Verification items for the finished model (mm, model axes). A direction names the side the tool comes from. Give positions to 0.01 mm unless a question says otherwise; leave off trailing zeros. Order: outer loops, then holes, each group sorted by start corner. A loop starts at its lowest first (then second) coordinate and runs counter-clockwise, first axis right, second up. Notation, with made-up numbers: (55.25, 0) -> (110.25, 0) arc R20 cw to (110.25, 33) -> close; hole circle Ø4 at (-6.75, 59). An arc over 180 degrees is marked (long way). One line per question, with ' | ' between items. Start each with the question number.
Q1. Section check A-A on x = 720. Record the cut outline in (y, z).
Q2. Access from +Z, -Z, +X, -X, +Y, -Y to the whole of each face (thin tool, end or side, straight path). Record for faces 3 (the flat face through (325.712, 4.93, -866.605)), 4 (the flat face through (869.54, 4.93, -1019.48)).
Q3. Go/stop test with flat-tipped pins: pin 1 (3 mm diameter, centred on x = 353.5, y = 7.5, fed in from +Z); pin 2 (5 mm diameter, centred on y = 4.5, z = -890.5, fed in from +X); pin 3 (6 mm diameter, centred on x = 1178, y = 9, fed in from -Z). Record where each tip stops, or that it passes through.
Q4. Section check D-D on x = 347. Record the cut outline in (y, z).
Q5. Material ranges on probe 1 along X at (y, z) = (7, -1119); probe 2 along X at (y, z) = (1.75, -945); probe 3 along Z at (x, y) = (1042, 5), recorded low to high. Write a range as [from, to].
Q6. Section check B-B on z = -682. Record the cut outline in (x, y).
Q7. Mould release check, pull along Z, two halves, no side actions. Record for faces 1 (the flat face through (745.285, 4.93, -1322.039)), 2 (the flat face through (611.047, 4.93, -1098.128)): released by +Z, released by -Z, zero draft, split by the parting line, or undercut.
Q8. Section check C-C on y = 7.25. Give the number of separate pieces and of enclosed holes in the cut face, plus the area to 3 significant figures.
from build123d import *

# Parameters (mm, degrees)
BOSS_EXTRUDE1_DEPTH = 10


with BuildPart() as part:
    # Sketch1 → Boss-Extrude1 (new body)
    with BuildSketch(Plane(origin=(0, 0, 0), x_dir=(1, 0, 0), z_dir=(0, 1, 0))):
        Polygon((784.987851723, 398.007183844), (785.000571871, 709.000734601), (783.999038632, 709.000734601), (648.95430554, 576.00627914), (204.012861183, 736.515465829), (389.346795443, 804.38206818), (260.269155542, 930.594602451), (438.985812263, 917.017059796), (281.997531244, 1251.994529906), (546.997134557, 1127.998293592), (540.820297596, 1358.942378927), (694.484658499, 1184.98269214), (797.527155209, 1462.988304378), (901.507891553, 1184.98269214), (1055.994737963, 1359.007597162), (1049.481640439, 1127.998293592), (1313.995431768, 1251.994529906), (1156.991756683, 916.99500763), (1334.998347933, 930.999939378), (1205.935810073, 803.988718502), (1391.001934492, 736.990931112), (946.559511347, 576.00627914), (810.545996287, 709.000734601), (809.987230906, 398.007183844), align=None)
        Polygon((768.211437064, 725.031722001), (643.992624095, 601.960316667), (269.679365999, 736.990931112), (486.122884579, 816.249412651), (530.047300467, 725.031722001), align=None, mode=Mode.SUBTRACT)
        Polygon((826.995686835, 725.031722001), (952.513065316, 601.960316667), (1325.302227186, 736.990931112), (1109.467295774, 816.249412651), (1065.831329223, 725.031722001), align=None, mode=Mode.SUBTRACT)
        Polygon((826.995686835, 747.043809063), (1052.054612149, 747.043809063), (1088.054253232, 823.06470125), (953.479995281, 872.126355119), align=None, mode=Mode.SUBTRACT)
        Polygon((767.95234015, 747.043809063), (543.908716076, 747.043809063), (507.909790164, 823.302917015), (642.157906737, 871.929882397), align=None, mode=Mode.SUBTRACT)
        Polygon((476.91056803, 836.361945246), (413.154674671, 813.015460537), (319.817787826, 904.533479576), (449.560148715, 894.676634268), align=None, mode=Mode.SUBTRACT)
        Polygon((1118.830884035, 836.361945246), (1182.869407152, 813.015460537), (1276.136882601, 903.669224766), (1146.140420035, 893.441560875), align=None, mode=Mode.SUBTRACT)
        Polygon((809.005952687, 760.999981232), (973.14510679, 924.891191926), (928.399604701, 1047.084725346), (809.005952687, 991.087402872), align=None, mode=Mode.SUBTRACT)
        Polygon((786.581669339, 760.999981232), (786.995069828, 991.087402872), (667.215871678, 1047.808759575), (622.403890172, 924.891191926), align=None, mode=Mode.SUBTRACT)
        Polygon((625.071199804, 890.100070463), (596.75349244, 919.234228308), (646.861936517, 1055.688427033), (328.365599037, 1206.51214806), (498.164892008, 844.477736382), align=None, mode=Mode.SUBTRACT)
        Polygon((970.890065096, 890.100070463), (1097.709804078, 843.529573856), (1267.828250082, 1206.51214806), (948.946832949, 1055.980771306), (999.021436359, 919.234228308), align=None, mode=Mode.SUBTRACT)
        Polygon((797.527155209, 1010.09324616), (920.701437633, 1068.238980962), (797.527155209, 1398.902304133), (674.967131634, 1068.238980962), align=None, mode=Mode.SUBTRACT)
        Polygon((654.433985107, 1077.890698346), (685.66424413, 1161.312305797), (564.365750317, 1299.115972687), (568.857249407, 1117.806751608), align=None, mode=Mode.SUBTRACT)
        Polygon((941.613316466, 1077.890698346), (1026.742088945, 1116.968977072), (1031.676560348, 1299.115972687), (910.781362362, 1160.123449622), align=None, mode=Mode.SUBTRACT)
    extrude(amount=BOSS_EXTRUDE1_DEPTH)


solid = part.part
Filled in:
1) outline: (0, -1253.82) -> (10, -1253.82) -> (10, -1189.74) -> (0, -1189.74) -> close; (0, -1046.87) -> (10, -1046.87) -> (10, -1022.81) -> (0, -1022.81) -> close; (0, -827.47) -> (10, -827.47) -> (10, -794.65) -> (0, -794.65) -> close; (0, -747.04) -> (10, -747.04) -> (10, -725.03) -> (0, -725.03) -> close; (0, -677.27) -> (10, -677.27) -> (10, -645.97) -> (0, -645.97) -> close
2) face 3: -X, +Y, -Y | face 4: +Y, -Y
3) pin 1: z = -682.05 | pin 2: x = 1296.38 | pin 3: z = -1189.65
4) outline: (0, -1221.58) -> (10, -1221.58) -> (10, -1197.69) -> (0, -1197.69) -> close; (0, -1166.78) -> (10, -1166.78) -> (10, -1113.29) -> (0, -1113.29) -> close; (0, -924.01) -> (10, -924.01) -> (10, -902.47) -> (0, -902.47) -> close; (0, -877.88) -> (10, -877.88) -> (10, -845.79) -> (0, -845.79) -> close; (0, -788.88) -> (10, -788.88) -> (10, -765.3) -> (0, -765.3) -> close; (0, -709.1) -> (10, -709.1) -> (10, -684.93) -> (0, -684.93) -> close
5) probe 1: [344.33, 369.41], [513.17, 568.83], [669.82, 693.78], [901.79, 926.2], [1026.8, 1082.44], [1226.81, 1251.67] | probe 2: [425.87, 451.02], [606.22, 629.73], [786.91, 809.01], [965.78, 989.59], [1145.27, 1170.12] | probe 3: [-1343.24, -1099.91], [-863.99, -839.85], [-747.04, -725.03], [-634.37, -610.58]
6) outline: (355.13, 0) -> (422.12, 0) -> (422.12, 10) -> (355.13, 10) -> close; (724.78, 0) -> (756.58, 0) -> (756.58, 10) -> (724.78, 10) -> close; (785, 0) -> (810.5, 0) -> (810.5, 10) -> (785, 10) -> close; (838.16, 0) -> (870.88, 0) -> (870.88, 10) -> (838.16, 10) -> close; (1173.48, 0) -> (1239.18, 0) -> (1239.18, 10) -> (1173.48, 10) -> close
7) face 1: released by -Z | face 2: undercut
8) separate pieces: 1 | enclosed holes: 13 | area: 187,000 mm²
